For this review, take the finished solid that the model builds, in its own axes (mm). A direction names the side the tool comes from. Coordinates: 2 decimals unless noted, no trailing zeros. Order: outer loops, then holes, each group sorted by start corner. A loop starts at its lowest first (then second) coordinate and runs counter-clockwise, first axis right, second up.
from build123d import *

# Parameters (mm, degrees)
BOSS_EXTRUDE1_DEPTH = 2.6
SKETCH2_R           = 1.5
BOSS_EXTRUDE2_DEPTH = 3
SKETCH6_R           = 1.5
BOSS_EXTRUDE3_DEPTH = 134
SKETCH8_R           = 1.5
CUT_EXTRUDE1_DEPTH  = 19.5
SKETCH9_R           = 1.5
CUT_EXTRUDE2_DEPTH  = 7
SKETCH10_R          = 1.965
SKETCH10_R_2        = 2
CUT_EXTRUDE4_DEPTH  = 0.5


with BuildPart() as part:
    # Sketch1 → Boss-Extrude1 (new body)
    with BuildSketch(Plane(origin=(0, 0, 0), x_dir=(1, 0, 0), z_dir=(0, 1, 0))):
        Polygon((-8.2, -7.407073571), (-8.2, -3.5), (-8.2, 0.15), (-5, 0.15), (-1.8, 0.15), (-1.8, -3.5), (-1.8, -7.407073571), (10.185852857, -7.407073571), (10.185852857, 3.5), (10.185852857, 7.592926429), (8.2, 7.592926429), (8.2, 3.5), (8.2, -0.15), (5, -0.15), (1.8, -0.15), (1.8, 3.5), (1.8, 7.592926429), (-9.814147143, 7.592926429), (-9.814147143, -7.407073571), align=None)
    extrude(amount=BOSS_EXTRUDE1_DEPTH)

    # Sketch2 → Boss-Extrude2 (add)
    with BuildSketch(Plane.XZ):
        Polygon((-8.2, 7.407073571), (-9.814147143, 7.407073571), (-9.814147143, -7.592926429), (1.8, -7.592926429), (1.8, -3.5), (1.8, 0.15), (5, 0.15), (8.2, 0.15), (8.2, -3.5), (8.2, -7.592926429), (10.185852857, -7.592926429), (10.185852857, -3.5), (10.185852857, 7.407073571), (-1.8, 7.407073571), (-1.8, 3.5), (-1.8, -0.15), (-5, -0.15), (-8.2, -0.15), (-8.2, 3.5), align=None)
        Polygon((1.8, -3.5), (1.8, -7.592926429), (5.185852857, -7.592926429), (8.2, -7.592926429), (8.2, -3.5), (8.2, 0.15), (5, 0.15), (1.8, 0.15), align=None)
        with Locations((5, -3.5)):
            Circle(SKETCH2_R, mode=Mode.SUBTRACT)
        Polygon((-1.8, 7.407073571), (-8.2, 7.407073571), (-8.2, 3.5), (-8.2, -0.15), (-5, -0.15), (-1.8, -0.15), (-1.8, 3.5), align=None)
        with Locations((-5, 3.5)):
            Circle(SKETCH2_R, mode=Mode.SUBTRACT)
    extrude(amount=BOSS_EXTRUDE2_DEPTH)

    # Sketch6 → Boss-Extrude3 (add)
    with BuildSketch(Plane(origin=(0, 2.6, 0), x_dir=(1, 0, 0), z_dir=(0, 1, 0))):
        Polygon((-8.2, -3.5), (-8.2, -7.407073571), (-1.8, -7.407073571), (-1.8, -3.5), (-1.8, 0.15), (-5, 0.15), (-8.2, 0.15), align=None)
        with Locations((-5, -3.5)):
            Circle(SKETCH6_R, mode=Mode.SUBTRACT)
        Polygon((5.185852857, 7.592926429), (1.8, 7.592926429), (1.8, 3.5), (1.8, -0.15), (5, -0.15), (8.2, -0.15), (8.2, 3.5), (8.2, 7.592926429), align=None)
        with Locations((5, 3.5)):
            Circle(SKETCH6_R, mode=Mode.SUBTRACT)
        Polygon((1.8, 7.592926429), (-9.814147143, 7.592926429), (-9.814147143, -7.407073571), (-8.2, -7.407073571), (-8.2, -3.5), (-8.2, 0.15), (-5, 0.15), (-1.8, 0.15), (-1.8, -3.5), (-1.8, -7.407073571), (10.185852857, -7.407073571), (10.185852857, 3.5), (10.185852857, 7.592926429), (8.2, 7.592926429), (8.2, 3.5), (8.2, -0.15), (5, -0.15), (1.8, -0.15), (1.8, 3.5), align=None)
        with Locations((-5, -3.5)):
            Circle(SKETCH6_R)
        with Locations((5, 3.5)):
            Circle(SKETCH6_R)
    extrude(amount=BOSS_EXTRUDE3_DEPTH)

    # Sketch8 → Cut-Extrude1 (cut)
    with BuildSketch(Plane.XZ.offset(3)):
        with Locations((-5, 3.5)):
            Circle(SKETCH8_R)
        with Locations((5, -3.5)):
            Circle(SKETCH8_R)
    extrude(amount=-CUT_EXTRUDE1_DEPTH, mode=Mode.SUBTRACT)

    # Sketch9 → Cut-Extrude2 (cut)
    with BuildSketch(Plane(origin=(0, 136.6, 0), x_dir=(1, 0, 0), z_dir=(0, 1, 0))):
        with Locations((-4.814147143, 0.092926429)):
            Circle(SKETCH9_R)
        with Locations((5.185852857, 0.092926429)):
            Circle(SKETCH9_R)
    extrude(amount=-CUT_EXTRUDE2_DEPTH, mode=Mode.SUBTRACT)

    # Sketch10 → Cut-Extrude4 (cut)
    with BuildSketch(Plane(origin=(0, 136.6, 0), x_dir=(1, 0, 0), z_dir=(0, 1, 0))):
        with Locations((-4.814147143, 0.092926429)):
            Circle(SKETCH10_R)
        with Locations((5.185852857, 0.092926429)):
            Circle(SKETCH10_R_2)
    extrude(amount=-CUT_EXTRUDE4_DEPTH, mode=Mode.SUBTRACT)


solid = part.part
1. Take a section at B-B, the plane z = -3.5. Give the boundary of the cut face in (x, y), plus the area to 3 significant figures.
Answer below:
outline: (-9.81, -3) - (3.5, -3) - (3.5, 0) - (1.8, 0) - (1.8, 2.6) - (3.5, 2.6) - (3.5, 16.5) - (6.5, 16.5) - (6.5, 2.6) - (8.2, 2.6) - (8.2, 0) - (6.5, 0) - (6.5, -3) - (10.19, -3) - (10.19, 136.6) - (-9.81, 136.6) - close
area: 2,720 mm2
2. Machinability: for faces 1 (the face through (6.57, 132.9, 0.48)), 2 (the face through (5, 1, 0.15)), 3 (the face through (-6.2, 9.5, 2.6)), which of the approach directions +Z, -Z, +X, -X, +Y, -Y give a long, thin tool a straight path to every point of the face, cutting with its end or side? Answer none if there is none.
Answer below:
face 1: +Y
face 2: -Z
face 3: -Y
3. Clearance check with flat-ended pins moving along their axes: pin 1 Ø1.3 at (x, y) = (4.5, 1.5) entering from -Z; pin 2 Ø0.9 at (x, z) = (-5, 0) entering from +Y; pin 3 Ø1.5 at (x, z) = (-5.5, 4) entering from -Y. State where each tip first meets the part, or that it passes through.
Answer below:
pin 1: stops at z = 0.15
pin 2: stops at y = 129.6
pin 3: stops at y = 16.5
4. To check wall thickness, follow L1, parallel to Y at x = 4, z = -5.25; L2, parallel to Z at x = -5, y = -2.1; L3, parallel to Z at x = 5, y = 9.25. State the ranges of each line that lie inside material, in increasing order.
Answer below:
L1: y = -3 to 0, 2.6 to 136.6
L2: z = -7.59 to 2, 5 to 7.41
L3: z = -7.59 to -5, -2 to 7.41
5. The part is to be moulded in two halves that separate along X. For faces 4 (the face through (-9.814, 66, 0)), 5 (the face through (10.186, 66, 0)), 6 (the face through (1.8, 1, -4)), say which applies: +X half, -X half, draft (parallel to the pull), parting line (faces both ways), or undercut.
Answer below:
face 4: -X half
face 5: +X half
face 6: undercut
6. Take a section at D-D, the plane x = -5. Give the boundary of the cut face in (y, z).
Answer below:
outline: (-3, -7.59) - (136.6, -7.59) - (136.6, -2.05) - (136.1, -2.05) - (136.1, -1.58) - (129.6, -1.58) - (129.6, 1.4) - (136.1, 1.4) - (136.1, 1.86) - (136.6, 1.86) - (136.6, 7.41) - (2.6, 7.41) - (2.6, 5) - (16.5, 5) - (16.5, 2) - (2.6, 2) - (2.6, -0.15) - (0, -0.15) - (0, 2) - (-3, 2) - close; (-3, 5) - (0, 5) - (0, 7.41) - (-3, 7.41) - close
7. Take a section at C-C, the plane y = 14.5. Give the boundary of the cut face in (x, z).
Answer below:
outline: (-9.81, -7.59) - (10.19, -7.59) - (10.19, 7.41) - (-9.81, 7.41) - close; hole circle Ø3 at (-5, 3.5); hole circle Ø3 at (5, -3.5)
8. Take a section at A-A, the plane x = 5. Give the boundary of the cut face in (y, z).
Answer below:
outline: (-3, -7.59) - (0, -7.59) - (0, -5) - (-3, -5) - close; (-3, -2) - (0, -2) - (0, 0.15) - (2.6, 0.15) - (2.6, -2) - (16.5, -2) - (16.5, -5) - (2.6, -5) - (2.6, -7.59) - (136.6, -7.59) - (136.6, -2.08) - (136.1, -2.08) - (136.1, -1.58) - (129.6, -1.58) - (129.6, 1.4) - (136.1, 1.4) - (136.1, 1.9) - (136.6, 1.9) - (136.6, 7.41) - (-3, 7.41) - close
